```python
from build123d import *

# Parameters (mm, degrees)
CROQUIS1_W              = 200
CROQUIS1_H              = 200
CROQUIS1_R              = 2.5
SALIENTE_EXTRUIR1_DEPTH = 4
CROQUIS2_W              = 158
CROQUIS2_H              = 158
CORTAR_EXTRUIR1_DEPTH   = 10
CROQUIS3_W              = 161
CROQUIS3_H              = 161
CORTAR_EXTRUIR2_DEPTH   = 10


with BuildPart() as part:
    # Croquis1 → Saliente-Extruir1 (new body)
    with BuildSketch(Plane(origin=(0, 0, 0), x_dir=(1, 0, 0), z_dir=(0, 1, 0))):
        with Locations((100, 100)):
            Rectangle(CROQUIS1_W, CROQUIS1_H)
        with Locations(Location((15, 185, 0), (0, 0, 270))):
            Circle(CROQUIS1_R, mode=Mode.SUBTRACT)
        with Locations(Location((185, 185, 0), (0, 0, 270))):
            Circle(CROQUIS1_R, mode=Mode.SUBTRACT)
        with Locations(Location((185, 15, 0), (0, 0, 270))):
            Circle(CROQUIS1_R, mode=Mode.SUBTRACT)
        with Locations(Location((15, 15, 0), (0, 0, 270))):
            Circle(CROQUIS1_R, mode=Mode.SUBTRACT)
    extrude(amount=SALIENTE_EXTRUIR1_DEPTH)

    # Croquis2 → Cortar-Extruir1 (cut)
    with BuildSketch(Plane(origin=(0, 4, 0), x_dir=(1, 0, 0), z_dir=(0, 1, 0))):
        with Locations((100, 100)):
            Rectangle(CROQUIS2_W, CROQUIS2_H)
    extrude(amount=-CORTAR_EXTRUIR1_DEPTH, mode=Mode.SUBTRACT)

    # Croquis3 → Cortar-Extruir2 (cut)
    with BuildSketch(Plane(origin=(0, 4, 0), x_dir=(1, 0, 0), z_dir=(0, 1, 0))):
        with Locations((100, 100)):
            Rectangle(CROQUIS3_W, CROQUIS3_H)
    extrude(amount=-CORTAR_EXTRUIR2_DEPTH, mode=Mode.SUBTRACT)


solid = part.part
```
Model file for the job. Use its own axes, mm. Give positions to 0.01 mm unless a question says otherwise; leave off trailing zeros. Write each loop counter-clockwise with the first axis right and the second up, starting at its lowest first coordinate (ties: lowest second). Pieces come first, ordered by that corner, then holes. Notation, with made-up numbers: M 74.5,-35 L 100.5,-35 A20 cw 100.5,-18 Z; hole C -33,-37 d7. An arc over 180 degrees is marked long. Use a Markdown table: item, result.
1) Cut at B-B (z = -99). List the corners of the cut face in (x, y).
Responses:
| item | result |
|---|---|
| outline | M 0,0 L 19.5,0 L 19.5,4 L 0,4 Z; M 180.5,0 L 200,0 L 200,4 L 180.5,4 Z |
2) Drill centre lines: line 1 (Z direction, x = 185, y = 2.9); line 2 (Z direction, x = 15.5, y = 2); line 3 (X direction, y = 3.1, z = -185). Where is each one in solid material? Low to high. Write a range as from..to.
Responses:
| item | result |
|---|---|
| line 1 | z = -200..-187.5, -182.5..-17.5, -12.5..0 |
| line 2 | z = -200..-187.45, -182.55..-17.45, -12.55..0 |
| line 3 | x = 0..12.5, 17.5..182.5, 187.5..200 |
3) Pin check, flat tip, straight feed: pin 1 (8 mm diameter, centred on x = 15, z = -185, fed in from -Y). Stop position of the tip, or through.
Responses:
| item | result |
|---|---|
| pin 1 | stops at y = 0 |
4) Cut at D-D (z = -15). List the corners of the cut face in (x, y), and give its area (3 significant figures).
Responses:
| item | result |
|---|---|
| outline | M 0,0 L 12.5,0 L 12.5,4 L 0,4 Z; M 17.5,0 L 182.5,0 L 182.5,4 L 17.5,4 Z; M 187.5,0 L 200,0 L 200,4 L 187.5,4 Z |
| area | 760 mm2 |
5) Cut at C-C (x = 15). List the corners of the cut face in (y, z), and give its area (3 significant figures).
Responses:
| item | result |
|---|---|
| outline | M 0,-200 L 4,-200 L 4,-187.5 L 0,-187.5 Z; M 0,-182.5 L 4,-182.5 L 4,-17.5 L 0,-17.5 Z; M 0,-12.5 L 4,-12.5 L 4,0 L 0,0 Z |
| area | 760 mm2 |
6) Cut at A-A (x = 40). List the corners of the cut face in (y, z).
Responses:
| item | result |
|---|---|
| outline | M 0,-200 L 4,-200 L 4,-180.5 L 0,-180.5 Z; M 0,-19.5 L 4,-19.5 L 4,0 L 0,0 Z |
7) Pull direction Z, two halves, no side cores. Call faces 1 (the cylindrical face through (14.04, 1.97, -182.69)), 2 (the cylindrical face through (13.5, 2, -17)), 3 (the flat face through (187, 4, -101)): +Z half, -Z half, draft (parallel to the pull), parting line (faces both ways), or undercut.
Responses:
| item | result |
|---|---|
| face 1 | undercut |
| face 2 | undercut |
| face 3 | draft |
